from build123d import *

# Parameters (mm, degrees)
F0_R        = 23.5
F0_R_2      = 22
F1_DEPTH    = 2
F2_R        = 45
F2_R_2      = 23.5
F3_DEPTH    = 10
F4_R        = 35
F4_R_2      = 27.5
F5_DEPTH    = 6
F5_FACE_R   = 45
F5_FACE_R_2 = 35
F6_DEPTH    = 11
F7_R        = 2
F8_DEPTH    = 21.001


with BuildPart() as f1:
    # F0 (on Top) → F1 (new body)
    with BuildSketch(Plane.XY):
        with Locations((10, 29.8)):
            Circle(F0_R)
        with Locations((10, 29.8)):
            Circle(F0_R_2, mode=Mode.SUBTRACT)
    extrude(amount=F1_DEPTH)

    # F2 (on face) → F3 (join)
    with BuildSketch(Plane.XY.offset(2)):
        with Locations((10, 29.8)):
            Circle(F2_R)
        with Locations((10, 29.8)):
            Circle(F2_R_2, mode=Mode.SUBTRACT)
    extrude(amount=-F3_DEPTH)

    # F4 (on face) → F5 (cut)
    with BuildSketch(Plane(origin=(0, 0, -8), x_dir=(1, 0, 0), z_dir=(0, 0, -1))):
        with Locations((10, -29.8)):
            Circle(F4_R)
        with Locations((10, -29.8)):
            Circle(F4_R_2, mode=Mode.SUBTRACT)
    extrude(amount=-F5_DEPTH, mode=Mode.SUBTRACT)

    # F5_face (on face) → F6 (join)
    with BuildSketch(Plane(origin=(10, 29.8, -8), x_dir=(1, 0, 0), z_dir=(0, 0, -1))):
        Circle(F5_FACE_R)
        Circle(F5_FACE_R_2, mode=Mode.SUBTRACT)
    extrude(amount=F6_DEPTH)

    # F7 (on face) → F8 (cut, through all)
    with BuildSketch(Plane(origin=(0, 0, -19), x_dir=(1, 0, 0), z_dir=(0, 0, -1))):
        with Locations((10, 10.2)):
            Circle(F7_R)
        with Locations((-30, -29.8)):
            Circle(F7_R)
        with Locations((10, -69.8)):
            Circle(F7_R)
        with Locations((50, -29.8)):
            Circle(F7_R)
    extrude(amount=-F8_DEPTH, mode=Mode.SUBTRACT)


solid = f1.part
Geometry: final body of the model. Coordinates: model frame, mm. A direction names the side the tool comes from. Round coordinates to 2 decimals unless told otherwise and drop trailing zeros. Write each loop counter-clockwise with the first axis right and the second up, starting at its lowest first coordinate (ties: lowest second). Pieces come first, ordered by that corner, then holes. Notation, with made-up numbers: M 8.5,-20.75 L 57.5,-20.75 A13 cw 57.5,-2.75 Z; hole C 60,49.25 d5. An arc over 180 degrees is marked long. Write item = value, one per line.
Item 1: Access query for faces 1 (the face through (-11, 48, -2)), 2 (the face through (9.74, 67.817, -8.647)). Directions: +Z, -Z, +X, -X, +Y, -Y. A direction counts if a zero-diameter tool reaches every point of the face in a straight line with its end or side. Return the directions, or none.
Findings:
face_1 = -Z
face_2 = +Z, -Z
Item 2: Section query A-A on x = 10. Return loops of the section in (y, z).
Findings:
outline = M -15.2,-19 L -12.2,-19 L -12.2,2 L -15.2,2 Z; M -8.2,-19 L -5.2,-19 L -5.2,-2 L 2.3,-2 L 2.3,-8 L 6.3,-8 L 6.3,0 L 7.8,0 L 7.8,2 L -8.2,2 Z; M 51.8,0 L 53.3,0 L 53.3,-8 L 57.3,-8 L 57.3,-2 L 64.8,-2 L 64.8,-19 L 67.8,-19 L 67.8,2 L 51.8,2 Z; M 71.8,-19 L 74.8,-19 L 74.8,2 L 71.8,2 Z
Item 3: Pin query (flat end, axial travel): P1, Ø3.5, axis at x = 50, y = 29.8, coming from the -Z side; P2, Ø6, axis at x = 43.5, z = -13, coming from the -Y side; P3, Ø12, axis at y = 12.5, z = -11.5, coming from the +X side; P4, Ø1.5, axis at x = 23, z = -4, coming from the -Y side. Return the tip coordinate at first contact, or that it passes through.
Findings:
P1 = through
P2 = -3.29
P3 = 53.56
P4 = -13.5
Item 4: Section query C-C on z = -13. Return loops of the section in (x, y), then the cut area to 3 significant figures.
Findings:
outline = C 10,29.8 d90; hole C -30,29.8 d4; hole C 10,29.8 d70; hole C 10,-10.2 d4; hole C 10,69.8 d4; hole C 50,29.8 d4
area = 2,460 mm^2
Item 5: Section query B-B on y = 29.8. Return loops of the section in (x, z), then the cut area to 3 significant figures.
Findings:
outline = M -35,-19 L -32,-19 L -32,2 L -35,2 Z; M -28,-19 L -25,-19 L -25,-2 L -17.5,-2 L -17.5,-8 L -13.5,-8 L -13.5,0 L -12,0 L -12,2 L -28,2 Z; M 32,0 L 33.5,0 L 33.5,-8 L 37.5,-8 L 37.5,-2 L 45,-2 L 45,-19 L 48,-19 L 48,2 L 32,2 Z; M 52,-19 L 55,-19 L 55,2 L 52,2 Z
area = 398 mm^2
Item 6: Material intervals for line 1 along X through (y, z) = (29.8, -11.5); line 2 along Y through (x, z) = (10, -6.25); line 3 along Y through (x, z) = (10, -10.75), sorted ascending. Write a range as [from, to].
Findings:
line_1 = [-35, -32], [-28, -25], [45, 48], [52, 55]
line_2 = [-15.2, -12.2], [-8.2, -5.2], [2.3, 6.3], [53.3, 57.3], [64.8, 67.8], [71.8, 74.8]
line_3 = [-15.2, -12.2], [-8.2, -5.2], [64.8, 67.8], [71.8, 74.8]
Item 7: Pull-direction query (Y, two-part tool) for faces 3 (the face through (33.1, 56.3, -19)), 4 (the face through (9.74, -12.183, -8.647)), 5 (the face through (0.24, 73.73, -8.35)); classes: pulls with the +Y half, pulls with the -Y half, needs draft (parallel to the pull), parting line crosses it, or undercut.
Findings:
face_3 = needs draft
face_4 = undercut
face_5 = parting line crosses it
Item 8: Section query D-D on x = -30. Return loops of the section in (y, z), then the cut area to 3 significant figures.
Findings:
outline = M 9.18,-19 L 27.8,-19 L 27.8,2 L 9.18,2 Z; M 31.8,-19 L 50.42,-19 L 50.42,2 L 31.8,2 Z
area = 782 mm^2
